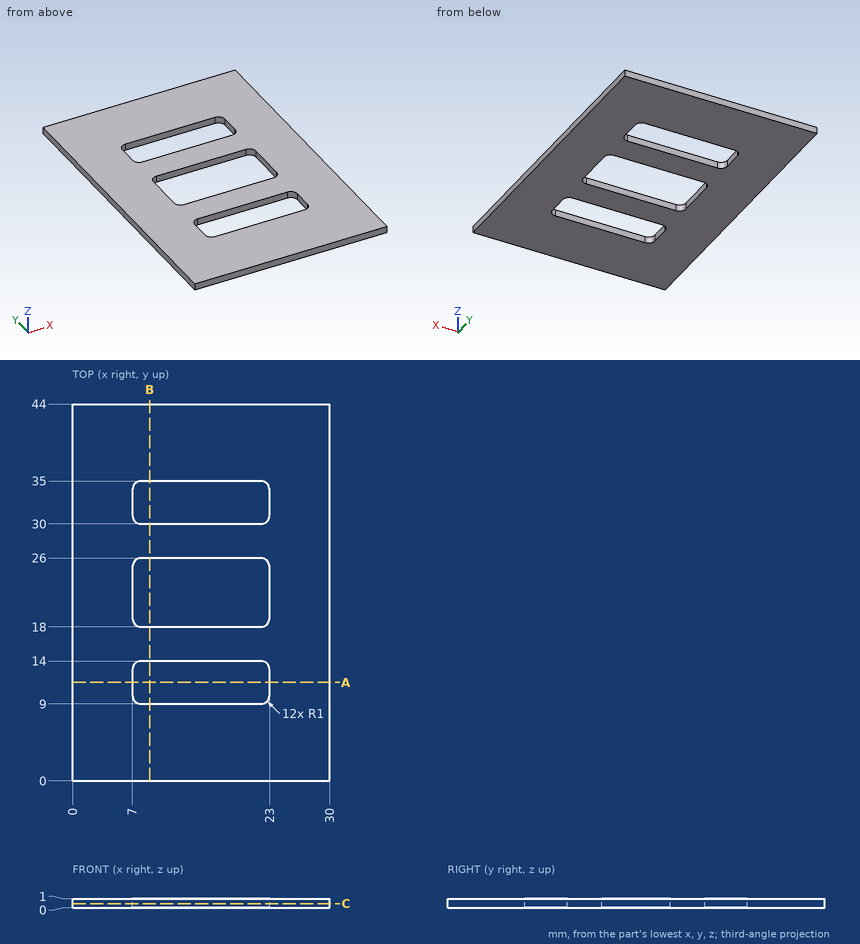
Geometry check sheet. Reference: drawing and pictorial views, mm from the part's lowest x, y, z. Round coordinates to 2 decimals unless told otherwise and drop trailing zeros. Write each loop counter-clockwise with the first axis right and the second up, starting at its lowest first coordinate (ties: lowest second). Pieces come first, ordered by that corner, then holes. Notation, with made-up numbers: (-39, 49.25) -> (-27, 49.25) arc R17 ccw to (-27, 70.25) -> close; hole circle Ø2 at (22.5, -26). An arc over 180 degrees is marked (long way). One line per question, with ' | ' between items. Start each with the question number.
1. Scan lines: line 1 along Y through (x, z) = (20, 0.7); line 2 along X through (y, z) = (33.5, 0.75); line 3 along Y through (x, z) = (22.5, 0.5). Record each from-to range of solid material in increasing order. Write a range as from..to.
2. Sectioned sample at B-B, the plane x = 9. Record the cut outline in (y, z), then the cut area to 3 significant figures.
3. Sectioned sample at C-C, the plane z = 0.45. Record the cut outline in (x, y).
4. Sectioned sample at A-A, the plane y = 11.5. Record the cut outline in (x, z).
Taken from the geometry:
1) line 1: y = 0..9, 14..18, 26..30, 35..44 | line 2: x = 0..7, 23..30 | line 3: y = 0..9.13, 13.87..18.13, 25.87..30.13, 34.87..44
2) outline: (0, 0) -> (9, 0) -> (9, 1) -> (0, 1) -> close; (14, 0) -> (18, 0) -> (18, 1) -> (14, 1) -> close; (26, 0) -> (30, 0) -> (30, 1) -> (26, 1) -> close; (35, 0) -> (44, 0) -> (44, 1) -> (35, 1) -> close | area: 26.0 mm^2
3) outline: (0, 0) -> (30, 0) -> (30, 44) -> (0, 44) -> close; hole (7, 10) arc R1 ccw to (8, 9) -> (22, 9) arc R1 ccw to (23, 10) -> (23, 13) arc R1 ccw to (22, 14) -> (8, 14) arc R1 ccw to (7, 13) -> close; hole (7, 19) arc R1 ccw to (8, 18) -> (22, 18) arc R1 ccw to (23, 19) -> (23, 25) arc R1 ccw to (22, 26) -> (8, 26) arc R1 ccw to (7, 25) -> close; hole (7, 31) arc R1 ccw to (8, 30) -> (22, 30) arc R1 ccw to (23, 31) -> (23, 34) arc R1 ccw to (22, 35) -> (8, 35) arc R1 ccw to (7, 34) -> close
4) outline: (0, 0) -> (7, 0) -> (7, 1) -> (0, 1) -> close; (23, 0) -> (30, 0) -> (30, 1) -> (23, 1) -> close
